Verification items for the finished model (mm, model axes). A direction names the side the tool comes from. Round coordinates to 2 decimals unless told otherwise and drop trailing zeros. Write each loop counter-clockwise with the first axis right and the second up, starting at its lowest first coordinate (ties: lowest second). Pieces come first, ordered by that corner, then holes.
from build123d import *

# Parameters (mm, degrees)
CROQUIS1_W              = 900
CROQUIS1_H              = 1047
SALIENTE_EXTRUIR1_DEPTH = 2113
VACIADO2_T              = -10
CROQUIS2_W              = 880
CROQUIS2_H              = 2093
SALIENTE_EXTRUIR2_DEPTH = 5
SALIENTE_EXTRUIR3_DEPTH = 300
CORTAR_EXTRUIR1_DEPTH   = 1044


with BuildPart() as part:
    # Croquis1 → Saliente-Extruir1 (new body)
    with BuildSketch(Plane(origin=(0, 0, 0), x_dir=(1, 0, 0), z_dir=(0, 1, 0))):
        Rectangle(CROQUIS1_W, CROQUIS1_H)
    extrude(amount=SALIENTE_EXTRUIR1_DEPTH)

    # Vaciado2
    vaciado2_openings = [part.faces().sort_by_distance(p)[0] for p in [
        (0, 1056.5, 523.5),
    ]]
    offset(amount=VACIADO2_T, openings=vaciado2_openings, kind=Kind.INTERSECTION)

    # Croquis2 → Saliente-Extruir2 (add)
    with BuildSketch(Plane.XY.offset(523.5)):
        with Locations((0, 1056.5)):
            Rectangle(CROQUIS2_W, CROQUIS2_H)
    extrude(amount=-SALIENTE_EXTRUIR2_DEPTH)

    # Croquis4 → Saliente-Extruir3 (add)
    with BuildSketch(Plane.XZ):
        with BuildLine():
            Line((-454.35645152, 548.5), (454.35645152, 548.5))
            ThreePointArc((454.35645152, 548.5), (468.953644638, 542.453644638), (475, 527.85645152))
            Line((475, 527.85645152), (475, -527.85645152))
            ThreePointArc((475, -527.85645152), (468.953644638, -542.453644638), (454.35645152, -548.5))
            Line((454.35645152, -548.5), (-454.35645152, -548.5))
            ThreePointArc((-454.35645152, -548.5), (-468.953644638, -542.453644638), (-475, -527.85645152))
            Line((-475, -527.85645152), (-475, 527.85645152))
            ThreePointArc((-475, 527.85645152), (-468.953644638, 542.453644638), (-454.35645152, 548.5))
        make_face()
    extrude(amount=SALIENTE_EXTRUIR3_DEPTH)

    # Croquis5 → Cortar-Extruir1 (cut)
    with BuildSketch(Plane.XY.offset(-513.5)):
        Polygon((-447, 10), (-447, 2110), (447, 2110), (447, 10), (447, 3), (-447, 3), align=None)
    extrude(amount=CORTAR_EXTRUIR1_DEPTH, mode=Mode.SUBTRACT)


solid = part.part
Q1. Depth check by flat-ended pin: P1, Ø10, axis at y = 1709, z = 93.5, coming from the -X side; P2, Ø12, axis at x = 56.5, y = 1023, coming from the +Z side; P3, Ø3, axis at y = 1542, z = 86, coming from the +X side. Enter the tip coordinate at first touch or a pass-through.
Recorded:
P1: stops at x = -450
P2: stops at z = -513.5
P3: stops at x = 450
Q2. Material ranges on line 1 along Y through (x, z) = (30.5, -131); line 2 along X through (y, z) = (1987, -340.5); line 3 along Z through (x, y) = (421.5, 1228), recorded low to high.
Recorded:
line 1: y = -300 to 3, 2110 to 2113
line 2: x = -450 to -447, 447 to 450
line 3: z = -523.5 to -513.5
Q3. Sectioned sample at B-B (y = 1305). Enter the section's corners in (x, z), plus the area to 3 significant figures.
Recorded:
outline: (-450, -523.5) - (450, -523.5) - (450, 523.5) - (447, 523.5) - (447, -513.5) - (-447, -513.5) - (-447, 523.5) - (-450, 523.5) - close
area: 15,200 mm2
Q4. Release check for a two-part mould opening along X. For faces 4 (the flat face through (6, 3, -2)), 5 (the flat face through (460, 0, 3)), 6 (the flat face through (-6, 2110, -2)), 7 (the flat face through (475, -148, 7)) record: released by +X, released by -X, zero draft, split by the parting line, or undercut.
Recorded:
face 4: undercut
face 5: zero draft
face 6: undercut
face 7: released by +X
Q5. Tool access check on faces 1 (the flat face through (-450, 1042, 7)), 2 (the flat face through (450, 1042, 7)), 3 (the flat face through (6, 1071, -513.5)). Record the directions out of +Z, -Z, +X, -X, +Y, -Y that give a thin tool (end or side, any length) a straight path to the whole face; none if there is none.
Recorded:
face 1: +Z, -Z, -X, +Y
face 2: +Z, -Z, +X, +Y
face 3: +Z
Q6. Sectioned sample at C-C (x = -288.5). Enter the section's corners in (y, z).
Recorded:
outline: (-300, -548.5) - (0, -548.5) - (0, -523.5) - (2113, -523.5) - (2113, 523.5) - (2110, 523.5) - (2110, -513.5) - (3, -513.5) - (3, 523.5) - (0, 523.5) - (0, 548.5) - (-300, 548.5) - close
Q7. Sectioned sample at A-A (z = 3). Enter the section's corners in (x, y).
Recorded:
outline: (-475, -300) - (475, -300) - (475, 0) - (450, 0) - (450, 2113) - (-450, 2113) - (-450, 0) - (-475, 0) - close; hole (-447, 3) - (447, 3) - (447, 2110) - (-447, 2110) - close
